```python
from build123d import *

# Parameters (mm, degrees)
BOSS_EXTRUDE2_DEPTH = 6.35
CIRPATTERN1_COUNT   = 20


with BuildPart() as part:
    # Sketch4 → Boss-Extrude2 (new body)
    with BuildSketch(Plane.XY):
        with BuildLine():
            Line((21.169137334, 1.852059533), (18.927699264, 1.655959112))
            ThreePointArc((18.927699264, 1.655959112), (18.837452366, 2.479997652), (18.711347307, 3.299315376))
            Line((18.711347307, 3.299315376), (0, 0))
            Line((0, 0), (18.711347307, -3.299315376))
            ThreePointArc((18.711347307, -3.299315376), (18.837452366, -2.479997652), (18.927699264, -1.655959112))
            Line((18.927699264, -1.655959112), (21.169137334, -1.852059533))
            ThreePointArc((21.169137334, -1.852059533), (23.12724618, -1.744088061), (24.97620554, -1.090484684))
            ThreePointArc((24.97620554, -1.090484684), (25, 0), (24.97620554, 1.090484684))
            ThreePointArc((24.97620554, 1.090484684), (23.12724618, 1.744088061), (21.169137334, 1.852059533))
        make_face()
    boss_extrude2 = extrude(amount=BOSS_EXTRUDE2_DEPTH)

    # CirPattern1: Boss-Extrude2 ×20 about axis
    cirpattern1_axis = Axis((0, 0, 0), (0, 0, 1))
    for i in range(1, CIRPATTERN1_COUNT):
        add(boss_extrude2.rotate(cirpattern1_axis, i * 360 / CIRPATTERN1_COUNT))


solid = part.part
```
Geometry check sheet. Reference: the model listing, model coordinates, mm. A direction names the side the tool comes from. Round coordinates to 2 decimals unless told otherwise and drop trailing zeros. Loops run counter-clockwise (first coordinate to the right, second up) from the corner with the lowest first, then second, coordinate; pieces in that order, holes last. Notation, with made-up numbers: M 78.5,59.25 L 103.5,59.25 A8 ccw 103.5,72.25 Z; hole C 59.25,87.25 d5. An arc over 180 degrees is marked long. Return JSON: item names as keys, results as strings. Group by question number.
(1) Set-up check for faces 1 (the face through (-18.54, -7.87, 3.13)), 2 (the face through (4.53, 19.62, 3.13)), 3 (the face through (-19.594, -4.524, 3.131)), 4 (the face through (-4.53, -19.62, 3.13)), 5 (the face through (22.51, 5.475, 3.131)): record each of +Z, -Z, +X, -X, +Y, -Y from which the full face is reachable in a straight line by a thin tool's end or side.
(2) Section check A-A, the plane y = 22. Enter the section's corners in (x, z), and give its area (3 significant figures).
(3) Go/stop test with flat-tipped pins: pin 1 (2 mm diameter, centred on x = -14.5, z = 5, fed in from +Y); pin 2 (2 mm diameter, centred on y = -17.5, z = 4.5, fed in from +X). Record where each tip stops, or that it passes through.
(4) Scan lines: line 1 along Y through (x, z) = (-18, 4.5); line 2 along Y through (x, z) = (-20.5, 0.75); line 3 along X through (y, z) = (-21, 5). Record each from-to range of solid material in increasing order. Write a range as [from, to].
(5) Mould release check, pull along Y, two halves, no side actions. Record for faces 6 (the face through (-15.016, 17.71, 3.131)), 7 (the face through (-10.37, -17.26, 3.13)), 8 (the face through (-15, 20, 3)): pulls with the +Y half, pulls with the -Y half, needs draft (parallel to the pull), parting line crosses it, or undercut.
(6) Section check B-B, the plane y = -2.5. Enter the section's corners in (x, z), and give its area (3 significant figures).
Data:
{
 "1": {"face 1": "+Z, -Z", "face 2": "+Z, -Z, +Y", "face 3": "+Z, -Z, -X", "face 4": "+Z, -Z, -Y", "face 5": "+Z, -Z, +X"},
 "2": {"outline": "M -8.85,0 L -5.22,0 L -5.22,6.35 L -8.85,6.35 Z; M -1.87,0 L 1.87,0 L 1.87,6.35 L -1.87,6.35 Z; M 5.22,0 L 8.85,0 L 8.85,6.35 L 5.22,6.35 Z", "area": "69.9 mm²"},
 "3": {"pin 1": "y = 20.85", "pin 2": "x = 15.32"},
 "4": {"line 1": "[-15.14, -10.82], [-7.64, 7.64], [10.82, 15.14]", "line 2": "[-14.31, -13.18], [-8.62, -4.73], [-1.79, 1.79], [4.73, 8.62], [13.18, 14.31]", "line 3": "[-8.74, -4.86], [-1.84, 1.84], [4.86, 8.74]"},
 "5": {"face 6": "undercut", "face 7": "pulls with the -Y half", "face 8": "pulls with the +Y half"},
 "6": {"outline": "M -18.83,0 L 18.83,0 L 18.83,6.35 L -18.83,6.35 Z", "area": "239 mm²"}
}
